Can you work these out from the model? Positions are in its coordinate system, mm. Face numbers are marked on the shaded views. A direction names the side the tool comes from. Coordinates: 2 decimals unless noted, no trailing zeros. Order: outer loops, then holes, each group sorted by start corner. A loop starts at its lowest first (then second) coordinate and runs counter-clockwise, first axis right, second up. Notation, with made-up numbers: (-3.5, -1) -> (13.5, -1) arc R21 ccw to (13.5, 13) -> close; hole circle Ø3 at (64, 16.25). An arc over 180 degrees is marked (long way). Answer as CSV lines item,"result".
from build123d import *

# Parameters (mm, degrees)
BOSS_EXTRUDE1_DEPTH    = 15
SKETCH3_R              = 20
CUT_EXTRUDE1_DEPTH     = 99.994949366
SKETCH4_R              = 40
CUT_EXTRUDE2_DEPTH     = 18
M10_TAPPED_HOLE1_D     = 8.5
M10_TAPPED_HOLE1_DEPTH = 24.5
M10_TAPPED_HOLE1_TIP   = 4.25


with BuildPart() as part:
    # Sketch1 → Boss-Extrude1 (new, symmetric)
    with BuildSketch(Plane.XY):
        with BuildLine():
            Line((-50, 80), (-50, 0))
            ThreePointArc((-50, 0), (0, -50), (50, 0))
            Line((50, 0), (50, 80))
            Line((50, 80), (-50, 80))
        make_face()
    extrude(amount=BOSS_EXTRUDE1_DEPTH, both=True)

    # Sketch3 → Cut-Extrude1 (cut, through all)
    with BuildSketch(Plane.XY.offset(15)):
        Circle(SKETCH3_R)
    extrude(amount=-CUT_EXTRUDE1_DEPTH, mode=Mode.SUBTRACT)

    # Sketch4 → Cut-Extrude2 (cut)
    with BuildSketch(Plane.XY.offset(15)):
        Circle(SKETCH4_R)
    extrude(amount=-CUT_EXTRUDE2_DEPTH, mode=Mode.SUBTRACT)

    # M10 Tapped Hole1
    with Locations(Plane(origin=(-35, 80, 0), x_dir=(0, 0, 1), z_dir=(0, 1, 0))):
        with Locations((0, 0), (0, 70)):
            Hole(M10_TAPPED_HOLE1_D / 2, depth=M10_TAPPED_HOLE1_DEPTH)
            with Locations((0, 0, -(M10_TAPPED_HOLE1_DEPTH + M10_TAPPED_HOLE1_TIP / 2))):  # 90° drill point
                Cone(0, M10_TAPPED_HOLE1_D / 2, M10_TAPPED_HOLE1_TIP, mode=Mode.SUBTRACT)


solid = part.part
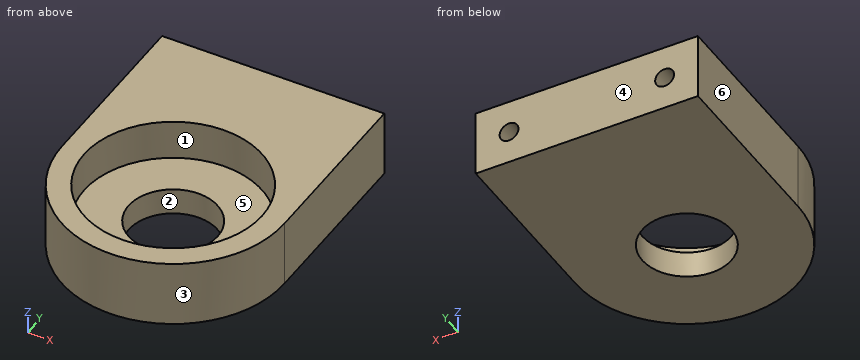
Q1. Imagine slicing it at A-A (x = 0). List the corners of the cut face in (y, z) for me.
Solution:
outline,"(-50, -15) -> (-20, -15) -> (-20, -3) -> (-40, -3) -> (-40, 15) -> (-50, 15) -> close; (20, -15) -> (80, -15) -> (80, 15) -> (40, 15) -> (40, -3) -> (20, -3) -> close"
Q2. Imagine slicing it at C-C (z = -11). List the corners of the cut face in (x, y) for me.
Solution:
outline,"(-50, 0) arc R50 ccw to (50, 0) -> (50, 80) -> (-50, 80) -> close; hole circle Ø40 at (0, 0)"
Q3. We'd pull the mould along X, two halves only. Please class the marked faces 1, 2, 3 and 4: pulls with the +X half, pulls with the -X half, needs draft (parallel to the pull), parting line crosses it, or undercut.
Solution:
face 1,"undercut"
face 2,"undercut"
face 3,"parting line crosses it"
face 4,"needs draft"
Q4. Imagine slicing it at D-D (y = -17.5). List the corners of the cut face in (x, z) for me.
Solution:
outline,"(-46.84, -15) -> (-9.68, -15) -> (-9.68, -3) -> (-35.97, -3) -> (-35.97, 15) -> (-46.84, 15) -> close; (9.68, -15) -> (46.84, -15) -> (46.84, 15) -> (35.97, 15) -> (35.97, -3) -> (9.68, -3) -> close"
Q5. Imagine slicing it at B-B (y = 62). List the corners of the cut face in (x, z) for me.
Solution:
outline,"(-50, -15) -> (50, -15) -> (50, 15) -> (-50, 15) -> close; hole circle Ø8.5 at (-35, 0); hole circle Ø8.5 at (35, 0)"
Q6. If I drill on line 1 (X direction, y = 69.5, z = 0); line 2 (Z direction, x = 35, y = 71.75); line 3 (Y direction, x = 0, z = -8.5), over which ranges is the centre line in solid material (lowest first)?
Solution:
line 1,"-50 to -39.25, -30.75 to 30.75, 39.25 to 50"
line 2,"-15 to -4.25, 4.25 to 15"
line 3,"-50 to -20, 20 to 80"
Q7. For P1, Ø7.5, axis at x = 35, z = 0, coming from the -Y side; P2, Ø5, axis at x = -35, z = 0, coming from the +Y side; P3, Ø3, axis at x = 1, y = -26.5, coming from the +Z side, each with a flat end and sliding along its axis, tell me the tip position at first contact or that it passes through.
Solution:
P1,"y = -39.03"
P2,"y = 53.75"
P3,"z = -3"
Q8. Which directions (+Z, -Z, +X, -X, +Y, -Y) give clear straight access to the entire face, cutting with the end or side of a thin tool? Please do the marked faces 5 and 6.
Solution:
face 5,"+Z"
face 6,"+Z, -Z, -X, +Y, -Y"
